The model under review builds one solid part; all positions refer to its coordinate system, in mm. Face numbers are marked on the shaded views. A direction names the side the tool comes from. Round coordinates to 2 decimals unless told otherwise and drop trailing zeros. Order: outer loops, then holes, each group sorted by start corner. A loop starts at its lowest first (then second) coordinate and runs counter-clockwise, first axis right, second up. Notation, with made-up numbers: M -9.5,46.25 L -0.5,46.25 A8 cw -0.5,57.25 Z; hole C 11,-27 d10. An arc over 180 degrees is marked long. Answer as a JSON object with one key per item and string values. Group by question number.
1. Add section D-D on y = 19. State the section outline as (x, z) points.
2. Add section A-A on z = 16. State the section outline as (x, y) points, and give its area (3 significant figures).
3. To check wall thickness, follow probe 1 along X at (y, z) = (0.6, 0); probe 2 along Y at (x, z) = (-4.5, -4); probe 3 along Z at (x, y) = (-1.5, 7.5). State the ranges of each line that lie inside material, in increasing order. Write a range as [from, to].
4. Mouldability with a two-part tool opening along Y and no side actions: class the marked faces 4, 5 and 6 as released by +Y, released by -Y, zero draft, split by the parting line, or undercut.
5. Clearance check with flat-ended pins moving along their axes: P1, Ø8, axis at y = 41, z = 4.5, coming from the -X side; P2, Ø1, axis at y = 0.5, z = 10, coming from the +X side; P3, Ø8, axis at y = 8, z = 1, coming from the +X side. State where each tip first meets the part, or that it passes through.
6. Machinability: for the marked faces 1, 2 and 3, which of the approach directions +Z, -Z, +X, -X, +Y, -Y give a long, thin tool a straight path to every point of the face, cutting with its end or side? Answer none if there is none.
7. Add section B-B on x = 0. State the section outline as (y, z) points.
8. Add section C-C on z = 0. State the section outline as (x, y) points.
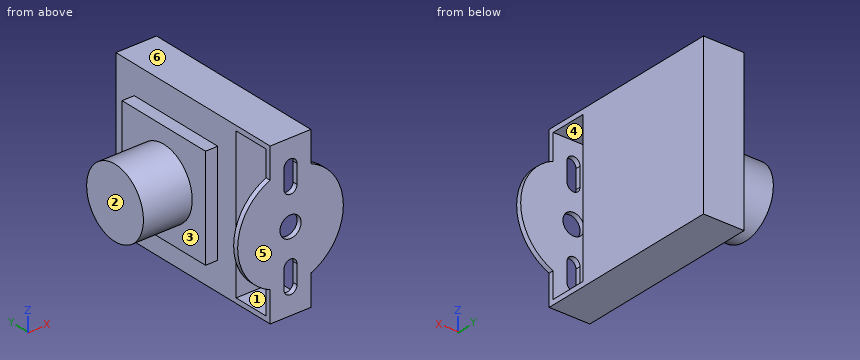
```python
from build123d import *

# Parameters (mm, degrees)
SKETCH_1_R          = 13
EXTRUDE_1_DEPTH     = 1.2
SKETCH_2_W          = 10
SKETCH_2_H          = 39
EXTRUDE_2_DEPTH     = 1.2
SKETCH_3_W          = 10
SKETCH_3_H          = 1.2
EXTRUDE_3_DEPTH     = 45
SKETCH_4_W          = 10
SKETCH_4_H          = 36
EXTRUDE_4_DEPTH     = 36.6
SKETCH_5_W          = 25
SKETCH_5_H          = 25
EXTRUDE_5_DEPTH     = 3
SKETCH_6_R          = 8.5
EXTRUDE_6_DEPTH     = 12
CUT_EXTRUDE_1_REACH = 55.988
SKETCH_7_R          = 2.6


with BuildPart() as part:
    # 草图1 → 凸台-拉伸1 (new body)
    with BuildSketch(Plane(origin=(0, 0, 0), x_dir=(1, 0, 0), z_dir=(0, 1, 0))):
        with Locations(Location((0, 0, 0), (0, 0, 270))):
            Circle(SKETCH_1_R)
    extrude(amount=EXTRUDE_1_DEPTH)

    # 草图2 → 凸台-拉伸2 (add)
    with BuildSketch(Plane(origin=(0, 1.2, 0), x_dir=(1, 0, 0), z_dir=(0, 1, 0))):
        Rectangle(SKETCH_2_W, SKETCH_2_H)
    extrude(amount=-EXTRUDE_2_DEPTH)

    # 草图3 → 凸台-拉伸3 (add)
    with BuildSketch(Plane(origin=(0, 1.2, 0), x_dir=(1, 0, 0), z_dir=(0, 1, 0))):
        with Locations((0, 18.9)):
            Rectangle(SKETCH_3_W, SKETCH_3_H)
    extrude_3 = extrude(amount=EXTRUDE_3_DEPTH)

    # 镜向1: 凸台-拉伸3 across plane
    add(extrude_3.mirror(Plane.XY))

    # 草图4 → 凸台-拉伸4 (add)
    with BuildSketch(Plane.XY.offset(-18.3)):
        with Locations((0, 28.2)):
            Rectangle(SKETCH_4_W, SKETCH_4_H)
    extrude(amount=EXTRUDE_4_DEPTH)

    # 草图5 → 凸台-拉伸5 (add)
    with BuildSketch(Plane.ZY.offset(5)):
        with Locations((0, 28.2)):
            Rectangle(SKETCH_5_W, SKETCH_5_H)
    extrude(amount=EXTRUDE_5_DEPTH)

    # 草图6 → 凸台-拉伸6 (add)
    with BuildSketch(Plane.ZY.offset(8)):
        with Locations((0, 28.2)):
            Circle(SKETCH_6_R)
    extrude(amount=EXTRUDE_6_DEPTH)

    # 草图7 → 切除-拉伸1 (cut, up to next)
    with BuildSketch(Plane.XZ, mode=Mode.PRIVATE) as cut_extrude_1_sk1:
        with Locations(Location((0, 0, 0), (0, 0, 270))):
            Circle(SKETCH_7_R)
    cut_extrude_1_tool1 = extrude(cut_extrude_1_sk1.sketch, amount=-CUT_EXTRUDE_1_REACH, mode=Mode.PRIVATE) & part.part
    # 草图7 → 切除-拉伸1 (cut, up to next)
    with BuildSketch(Plane.XZ, mode=Mode.PRIVATE) as cut_extrude_1_sk2:
        with BuildLine():
            Line((-1.6, 8.7), (-1.6, 13.3))
            ThreePointArc((-1.6, 13.3), (0, 14.9), (1.6, 13.3))
            Line((1.6, 13.3), (1.6, 8.7))
            ThreePointArc((1.6, 8.7), (0, 7.1), (-1.6, 8.7))
        make_face()
    cut_extrude_1_tool2 = extrude(cut_extrude_1_sk2.sketch, amount=-CUT_EXTRUDE_1_REACH, mode=Mode.PRIVATE) & part.part
    # 草图7 → 切除-拉伸1 (cut, up to next)
    with BuildSketch(Plane.XZ, mode=Mode.PRIVATE) as cut_extrude_1_sk3:
        with BuildLine():
            Line((-1.6, -8.7), (-1.6, -13.3))
            ThreePointArc((-1.6, -13.3), (0, -14.9), (1.6, -13.3))
            Line((1.6, -13.3), (1.6, -8.7))
            ThreePointArc((1.6, -8.7), (0, -7.1), (-1.6, -8.7))
        make_face()
    cut_extrude_1_tool3 = extrude(cut_extrude_1_sk3.sketch, amount=-CUT_EXTRUDE_1_REACH, mode=Mode.PRIVATE) & part.part
    add(cut_extrude_1_tool1.solids().sort_by_distance((0, 0, 0))[0], mode=Mode.SUBTRACT)
    add(cut_extrude_1_tool2.solids().sort_by_distance((0, 0, 11))[0], mode=Mode.SUBTRACT)
    add(cut_extrude_1_tool3.solids().sort_by_distance((0, 0, -11))[0], mode=Mode.SUBTRACT)


solid = part.part
```
Recorded:
{
 "1": {"outline": "M -8,-12.5 L -5,-12.5 L -5,-19.5 L 5,-19.5 L 5,19.5 L -5,19.5 L -5,12.5 L -8,12.5 Z"},
 "2": {"outline": "M -5,0 L 5,0 L 5,1.2 L -5,1.2 Z; M -5,10.2 L 5,10.2 L 5,46.2 L -5,46.2 Z", "area": "372 mm²"},
 "3": {"probe 1": "x = [-13, -2.6], [2.6, 13]", "probe 2": "y = [0, 1.2], [10.2, 46.2]", "probe 3": "z = [-19.5, -18.3], [18.3, 19.5]"},
 "4": {"face 4": "undercut", "face 5": "released by -Y", "face 6": "zero draft"},
 "5": {"P1": "stops at x = -8", "P2": "stops at x = 8.87", "P3": "stops at x = 5"},
 "6": {"face 1": "+X, -X", "face 2": "+Z, -Z, -X, +Y, -Y", "face 3": "-X"},
 "7": {"outline": "M 0,-19.5 L 46.2,-19.5 L 46.2,19.5 L 0,19.5 L 0,14.9 L 1.2,14.9 L 1.2,18.3 L 10.2,18.3 L 10.2,-18.3 L 1.2,-18.3 L 1.2,-14.9 L 0,-14.9 Z; M 0,-7.1 L 1.2,-7.1 L 1.2,-2.6 L 0,-2.6 Z; M 0,2.6 L 1.2,2.6 L 1.2,7.1 L 0,7.1 Z"},
 "8": {"outline": "M -20,19.7 L -8,19.7 L -8,15.7 L -5,15.7 L -5,10.2 L 5,10.2 L 5,46.2 L -5,46.2 L -5,40.7 L -8,40.7 L -8,36.7 L -20,36.7 Z; M -13,0 L -2.6,0 L -2.6,1.2 L -13,1.2 Z; M 2.6,0 L 13,0 L 13,1.2 L 2.6,1.2 Z"}
}
